Here's how the part is built. I have some questions about the finished solid (model axes, mm). Face numbers are marked on the shaded views. Coordinates: 2 decimals unless noted, no trailing zeros. Write each loop counter-clockwise with the first axis right and the second up, starting at its lowest first coordinate (ties: lowest second). Pieces come first, ordered by that corner, then holes.
Item 1: We'd pull the mould along X, two halves only. Please class the marked faces 1, 2, 3 and 4: +X half, -X half, draft (parallel to the pull), parting line (faces both ways), or undercut.
Item 2: If we section it at D-D (y = -47): Please give me the cut outline in (x, z).
Item 3: If we section it at C-C (z = 22): Please give me the cut outline in (x, y), then the cut area to 3 significant figures.
Item 4: If we section it at B-B (y = 87): Please give me the cut outline in (x, z).
Item 5: I'm going to push flat-ended pins straight in: pin 1 Ø1 at (x, y) = (29.5, 79.5) entering from +Z; pin 2 Ø6 at (x, z) = (-5.5, 19.5) entering from +Y; pin 3 Ø10 at (x, z) = (-3, 32) entering from -Y; pin 4 Ø11 at (x, y) = (0, 87) entering from +Z. Where does each tip first touch, or does it pass through?
Item 6: If I drill on line 1 (Y direction, x = -47, z = 3); line 2 (X direction, y = 23, z = 16); line 3 (Z direction, x = 9, y = 41), over which ranges is the centre line in solid material (lowest first)?
Item 7: If we section it at A-A (x = 47): Please give me the cut outline in (y, z).
from build123d import *

# Parameters (mm, degrees)
SKETCH1_W               = 124
SKETCH1_H               = 164
SKETCH1_R               = 6
BOSS_EXTRUDE1_DEPTH     = 5
BOSS_EXTRUDE2_DEPTH     = 55
CUT_EXTRUDE1_DEPTH      = 152.122466894
CUT_EXTRUDE1_DEPTH_BACK = 152.122466894


with BuildPart() as part:
    # Sketch1 → Boss-Extrude1 (new body)
    with BuildSketch(Plane.XY):
        with Locations((0, 20)):
            Rectangle(SKETCH1_W, SKETCH1_H)
        with Locations((0, 87)):
            Circle(SKETCH1_R, mode=Mode.SUBTRACT)
        with Locations((47, -47)):
            Circle(SKETCH1_R, mode=Mode.SUBTRACT)
        with Locations(Location((-47, -47, 0), (0, 0, 180))):
            Circle(SKETCH1_R, mode=Mode.SUBTRACT)
        with BuildLine():
            Line((35, 75), (35, 0))
            ThreePointArc((35, 0), (0, -35), (-35, 0))
            Line((-35, 0), (-35, 75))
            Line((-35, 75), (-30, 75))
            Line((-30, 75), (-30, 0))
            ThreePointArc((-30, 0), (0, -30), (30, 0))
            Line((30, 0), (30, 75))
            Line((30, 75), (35, 75))
        make_face(mode=Mode.SUBTRACT)
    extrude(amount=BOSS_EXTRUDE1_DEPTH)

    # Sketch1_2 → Boss-Extrude2 (add)
    with BuildSketch(Plane.XY):
        with BuildLine():
            Line((35, 0), (35, 75))
            Line((35, 75), (30, 75))
            Line((30, 75), (30, 0))
            ThreePointArc((30, 0), (21.213203436, -21.213203436), (0, -30))
            Line((0, -30), (0, -35))
            ThreePointArc((0, -35), (24.748737342, -24.748737342), (35, 0))
        make_face()
        with BuildLine():
            ThreePointArc((-35, 0), (-24.748737342, -24.748737342), (0, -35))
            Line((0, -35), (0, -30))
            ThreePointArc((0, -30), (-21.213203436, -21.213203436), (-30, 0))
            Line((-30, 0), (-30, 75))
            Line((-30, 75), (-35, 75))
            Line((-35, 75), (-35, 0))
        make_face()
    extrude(amount=BOSS_EXTRUDE2_DEPTH)

    # Sketch2 → Cut-Extrude1 (cut, two sides: drawn at the far end of the back side and taken through both)
    with BuildSketch(Plane(origin=(35, 0, 0), x_dir=(0, 0, -1), z_dir=(1, 0, 0)).offset(-CUT_EXTRUDE1_DEPTH_BACK)):
        Polygon((-55, 14), (-5, 75), (-55, 75), align=None)
    extrude(amount=CUT_EXTRUDE1_DEPTH + CUT_EXTRUDE1_DEPTH_BACK, mode=Mode.SUBTRACT)


solid = part.part
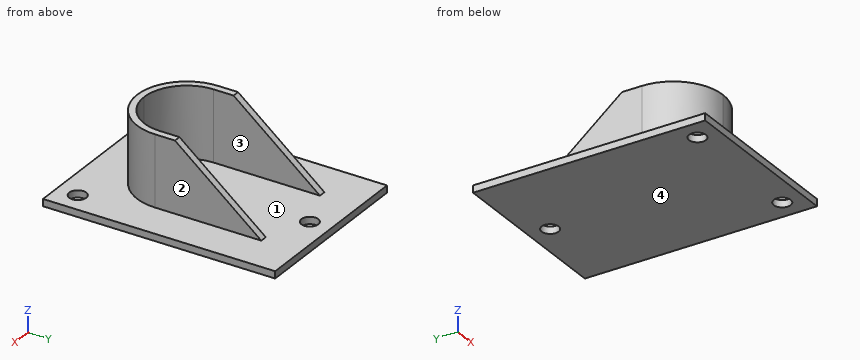
Answer list:
1. face 1: undercut
1. face 2: +X half
1. face 3: undercut
1. face 4: draft
2. outline: (-62, 0) - (-53, 0) - (-53, 5) - (-62, 5) - close; (-41, 0) - (41, 0) - (41, 5) - (-41, 5) - close; (53, 0) - (62, 0) - (62, 5) - (53, 5) - close
3. outline: (-35, 0) arc R35 ccw to (35, 0) - (35, 54.26) - (30, 54.26) - (30, 0) arc R30 cw to (-30, 0) - (-30, 54.26) - (-35, 54.26) - close
3. area: 1,050 mm2
4. outline: (-62, 0) - (-6, 0) - (-6, 5) - (-62, 5) - close; (6, 0) - (62, 0) - (62, 5) - (6, 5) - close
5. pin 1: stops at z = 5
5. pin 2: stops at y = -28.77
5. pin 3: stops at y = -35
5. pin 4: passes through
6. line 1: y = -62 to -53, -41 to 102
6. line 2: x = -35 to -30, 30 to 35
6. line 3: z = 0 to 5
7. outline: (-62, 0) - (-53, 0) - (-53, 5) - (-62, 5) - close; (-41, 0) - (102, 0) - (102, 5) - (-41, 5) - close
